Geometry check sheet. Reference: the model listing, model coordinates, mm. A direction names the side the tool comes from. Coordinates: 2 decimals unless noted, no trailing zeros. Order: outer loops, then holes, each group sorted by start corner. A loop starts at its lowest first (then second) coordinate and runs counter-clockwise, first axis right, second up. Notation, with made-up numbers: (29, -30.75) - (67, -30.75) arc R35 cw to (67, 8.25) - close; hole circle Ø4 at (31.5, -32). An arc over 180 degrees is marked (long way). Return JSON: item names as keys, results as strings. Group by question number.
Item 1: Scan lines: probe 1 along Z at (x, y) = (-2, 26); probe 2 along X at (y, z) = (13, -17); probe 3 along Z at (x, y) = (-14.5, 32.5). Record each from-to range of solid material in increasing order.
Item 2: Section check A-A on y = 3.5. Enter the section's corners in (x, z), then the cut area to 3 significant figures.
Item 3: Draft check along Z on faces 1 (the cylindrical face through (-23.048, 9.464, -120.148)), 2 (the flat face through (26.558, 26, -125)), 3 (the cylindrical face through (-14.79, 37.97, 125.5)), 4 (the flat face through (-26.055, 9, -2)). Enter one of: pulls with the +Z half, pulls with the -Z half, needs draft (parallel to the pull), parting line crosses it, or undercut.
Item 4: Tool access check on faces 5 (the cylindrical face through (-25.048, -0.986, -122.148)), 6 (the flat face through (6, 21, -127)), 7 (the flat face through (-2, 51.188, -1)). Record the directions out of +Z, -Z, +X, -X, +Y, -Y that give a thin tool (end or side, any length) a straight path to the whole face; none if there is none.
Item 5: Gauge pin test, flat ends, axial feed: pin 1 (2 mm diameter, centred on y = 30, z = -6, fed in from -X); pin 2 (0.6 mm diameter, centred on y = -1, z = -40.5, fed in from +X); pin 3 (1 mm diameter, centred on y = 49, z = 29.5, fed in from -X). Record the tip position at first contact, or that the pin passes through.
Item 6: Section check B-B on z = -51. Enter the section's corners in (x, y).
from build123d import *

# Parameters (mm, degrees)
SALIENTE_EXTRUIR1_DEPTH = 123
SALIENTE_EXTRUIR2_DEPTH = 4
CROQUIS3_W              = 2
CROQUIS3_H              = 4
CORTAR_EXTRUIR1_DEPTH   = 30.221833509
CROQUIS3_3_W            = 2
CROQUIS3_3_H            = 2
CORTAR_EXTRUIR2_DEPTH   = 54.613071269
REDONDEO2_R             = 10
REDONDEO3_R             = 5


# Read off the part's stored shape, not the designer's step: Simetría1
with BuildPart() as part:
    # Croquis1 → Saliente-Extruir1 (new, symmetric)
    with BuildSketch(Plane.XY):
        Polygon((-30.055424469, 20), (-30.055424469, 0), (-30.055424469, -2), (-28.055424469, -2), (-28.055424469, 0), (-26.055424469, 0), (-26.055424469, 18.666666667), (-1.66418671, 51.188317013), (-3.66418671, 51.188317013), (-3.66418671, 55.188317013), align=None)
    extrude(amount=SALIENTE_EXTRUIR1_DEPTH, both=True)

    # Croquis2 → Saliente-Extruir2 (add)
    with BuildSketch(Plane.XY.offset(123)):
        Polygon((26.5576468, 13.444650029), (26.5576468, 18.666666667), (26.5576468, 55.188317013), (-3.66418671, 55.188317013), (-30.055424469, 20), (-30.055424469, 14.33808094), (-30.055424469, -2), (26.5576468, -2), align=None)
    extrude(amount=SALIENTE_EXTRUIR2_DEPTH)

    # Croquis3 → Cortar-Extruir1 (cut)
    with BuildSketch(Plane(origin=(26.5576468, 0, 0), x_dir=(0, 0, -1), z_dir=(1, 0, 0))):
        with Locations((-124, 53.188317013)):
            Rectangle(CROQUIS3_W, CROQUIS3_H)
    extrude(amount=-CORTAR_EXTRUIR1_DEPTH, mode=Mode.SUBTRACT)

    # Croquis3<3> → Cortar-Extruir2 (cut)
    with BuildSketch(Plane(origin=(26.5576468, 0, 0), x_dir=(0, 0, -1), z_dir=(1, 0, 0))):
        with Locations((-124, -1)):
            Rectangle(CROQUIS3_3_W, CROQUIS3_3_H)
    extrude(amount=-CORTAR_EXTRUIR2_DEPTH, mode=Mode.SUBTRACT)

    # Redondeo2
    redondeo2_edges = [part.edges().sort_by_distance(p)[0] for p in [
        (-26.055424469, 9.333333333, 123),
        (-3.664186709, 53.188317013, 125),
        (-28.055424469, -1, 125),
        (-13.85980559, 34.92749184, 123),
    ]]
    fillet(redondeo2_edges, radius=REDONDEO2_R)

    # Redondeo3
    redondeo3_edges = [part.edges().sort_by_distance(p)[0] for p in [
        (-16.85980559, 37.594158506, 127),
        (-30.055424469, 9, 127),
    ]]
    fillet(redondeo3_edges, radius=REDONDEO3_R)

    # Simetría1
    split(bisect_by=Plane(origin=(0, 0, 0), x_dir=(1, 0, 0), z_dir=(0, 0, -1)), keep=Keep.BOTTOM)

    # Simetr_a1 2: part across plane


with BuildPart() as part_1:
    add(part.part)
    add(part.part.mirror(Plane(origin=(0, 0, 0), x_dir=(1, 0, 0), z_dir=(0, 0, -1))))


solid = part_1.part
Computed:
{
 "1": {"probe 1": "z = -127 to -123, 123 to 127", "probe 2": "x = -30.06 to -26.06", "probe 3": "z = -127 to -117.24, 117.24 to 127"},
 "2": {"outline": "(-30.06, -122) arc R5 ccw to (-25.06, -127) - (26.56, -127) - (26.56, -123) - (-16.06, -123) arc R10 cw to (-26.06, -113) - (-26.06, 113) arc R10 cw to (-16.06, 123) - (26.56, 123) - (26.56, 127) - (-25.06, 127) arc R5 ccw to (-30.06, 122) - close", "area": "1,470 mm²"},
 "3": {"face 1": "undercut", "face 2": "needs draft", "face 3": "pulls with the +Z half", "face 4": "undercut"},
 "4": {"face 5": "+X, -Y", "face 6": "-Z, +X, -X, +Y, -Y", "face 7": "+X, +Y"},
 "5": {"pin 1": "stops at x = -23.31", "pin 2": "stops at x = -28.06", "pin 3": "stops at x = -8.68"},
 "6": {"outline": "(-30.06, -2) - (-28.06, -2) - (-28.06, 0) - (-26.06, 0) - (-26.06, 18.67) - (-1.66, 51.19) - (-3.66, 51.19) - (-3.66, 55.19) - (-30.06, 20) - close"}
}
